from build123d import *

# Parameters (mm, degrees)
SKETCH1_R           = 14
BOSS_EXTRUDE1_DEPTH = 50


with BuildPart() as part:
    # Sketch1 → Boss-Extrude1 (new body)
    with BuildSketch(Plane.XY):
        with BuildLine():
            Line((0, 0), (-76.096455974, 0))
            Line((-76.096455974, 0), (-90.096455974, 14))
            Line((-90.096455974, 14), (-90.096455974, 50))
            Line((-90.096455974, 50), (-76.096455974, 64))
            Line((-76.096455974, 64), (-62.096455974, 64))
            Line((-62.096455974, 64), (-21.972137383, 56.92500005))
            ThreePointArc((-21.972137383, 56.92500005), (1.024616064, 60.067940114), (17.903544026, 76))
            Line((17.903544026, 76), (75.903544026, 76))
            Line((75.903544026, 76), (85.903544026, 66))
            Line((85.903544026, 66), (85.903544026, 18))
            Line((85.903544026, 18), (27.903544026, -38))
            Line((27.903544026, -38), (23.442882283, -38))
            ThreePointArc((23.442882283, -38), (14.564937889, -24.231344122), (9.891277483, -8.529411765))
            ThreePointArc((9.891277483, -8.529411765), (6.530471562, -2.426827536), (0, 0))
        make_face()
        with Locations((-62.096455974, 28)):
            Circle(SKETCH1_R, mode=Mode.SUBTRACT)
    extrude(amount=BOSS_EXTRUDE1_DEPTH)


solid = part.part
Build history of the part. All positions in model axes, mm. A direction names the side the tool comes from. Round coordinates to 2 decimals unless told otherwise and drop trailing zeros. Write each loop counter-clockwise with the first axis right and the second up, starting at its lowest first coordinate (ties: lowest second). Pieces come first, ordered by that corner, then holes. Notation, with made-up numbers: (68.25, 79) -> (111.25, 79) arc R33 ccw to (111.25, 112) -> close; hole circle Ø11 at (-29.75, 31). An arc over 180 degrees is marked (long way). Use one line per item in the form item = value.
Q1. Drop flat-ended pins along their axis: P1, Ø4, axis at x = -71, z = 14, coming from the +Y side; P2, Ø5, axis at x = -64.5, z = 19, coming from the -Y side. Give the stop position or say it passes through.
Conclusion:
P1 = 64
P2 = 0
Q2. Band-saw the part on A-A, the plane y = 28. Write the cut outline in (x, z).
Conclusion:
outline = (-90.1, 0) -> (-76.1, 0) -> (-76.1, 50) -> (-90.1, 50) -> close; (-48.1, 0) -> (85.9, 0) -> (85.9, 50) -> (-48.1, 50) -> close
Q3. Drill centre lines: L1, parallel to Y at x = 53, z = 17; L2, parallel to X at y = 26.5, z = 20; L3, parallel to X at y = -18, z = 34. Where is each one in solid material? Low to high.
Conclusion:
L1 = -13.77 to 76
L2 = -90.1 to -76.02, -48.18 to 85.9
L3 = 12.12 to 48.62
Q4. Band-saw the part on C-C, the plane x = 44.5. Write the cut outline in (y, z), then the cut area to 3 significant figures.
Conclusion:
outline = (-21.98, 0) -> (76, 0) -> (76, 50) -> (-21.98, 50) -> close
area = 4,900 mm²
Q5. Band-saw the part on B-B, the plane z = 39.5. Write the cut outline in (x, y) (1 decimal).
Conclusion:
outline = (-90.1, 14) -> (-76.1, 0) -> (0, 0) arc R10 cw to (9.9, -8.5) arc R58 ccw to (23.4, -38) -> (27.9, -38) -> (85.9, 18) -> (85.9, 66) -> (75.9, 76) -> (17.9, 76) arc R38 cw to (-22, 56.9) -> (-62.1, 64) -> (-76.1, 64) -> (-90.1, 50) -> close; hole circle Ø28 at (-62.1, 28)
Q6. Band-saw the part on D-D, the plane y = 10.5. Write the cut outline in (x, z), then the cut area to 3 significant figures.
Conclusion:
outline = (-86.6, 0) -> (78.14, 0) -> (78.14, 50) -> (-86.6, 50) -> close
area = 8,240 mm²
Q7. Tool access for faces 1 (the flat face through (-42.315, 60.512, 24.65)), 2 (the flat face through (-69, 64, 25)), 3 (the flat face through (-38, 0, 25)): list every direction of +Z, -Z, +X, -X, +Y, -Y with a clear straight run to the whole face (end or side of a thin tool).
Conclusion:
face_1 = +Z, -Z, +Y
face_2 = +Z, -Z, -X, +Y
face_3 = +Z, -Z, -X, -Y
